The drawing under review shows one solid part. Ordinate dimensions are in mm from its lowest x, y, z. A direction names the side the tool comes from. Give positions to 0.01 mm unless a question says otherwise; leave off trailing zeros. Loops run counter-clockwise (first coordinate to the right, second up) from the corner with the lowest first, then second, coordinate; pieces in that order, holes last. Notation, with made-up numbers: M -7,63.5 L 39,63.5 A26 ccw 39,80.5 Z; hole C -2.5,63 d6. An arc over 180 degrees is marked long. Answer as CSV lines item,"result".
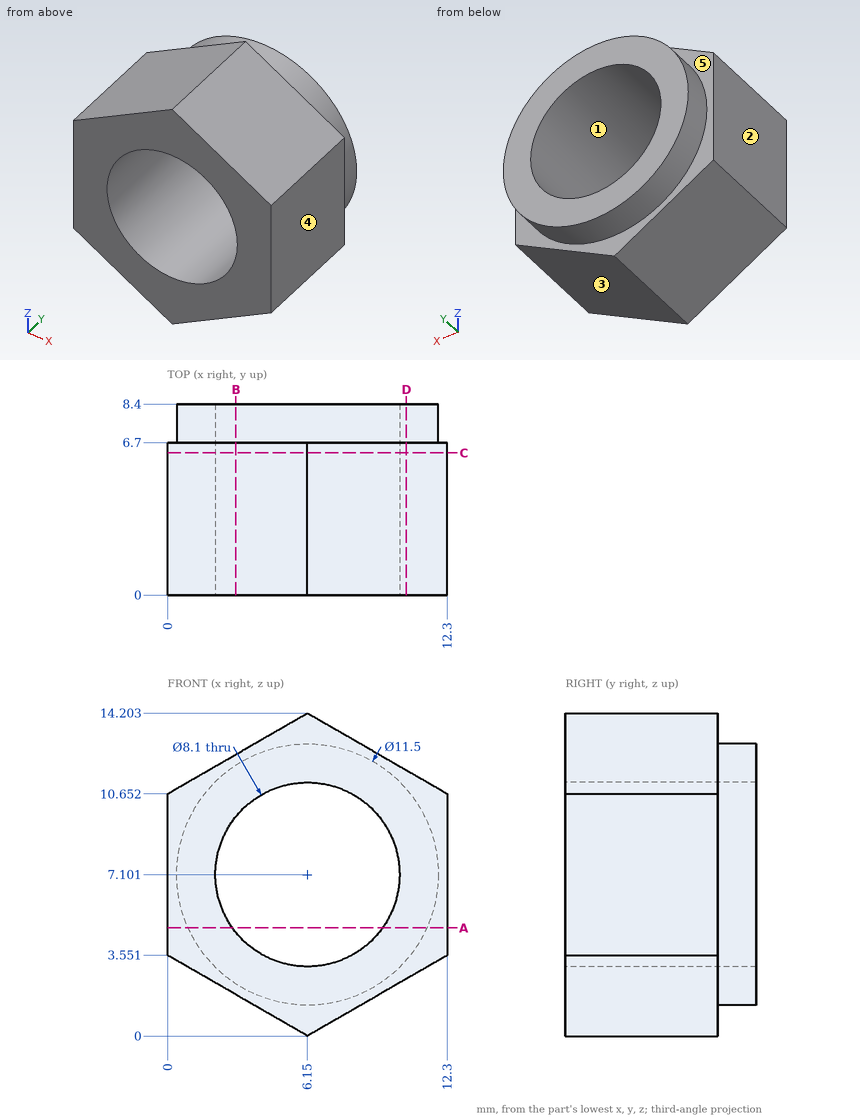
1. We need section B-B, the plane x = 3. Write out the cut boundary in (y, z) (1 decimal).
Answer block:
outline,"M 0,1.8 L 6.7,1.8 L 6.7,2.3 L 8.4,2.3 L 8.4,4.6 L 0,4.6 Z; M 0,9.6 L 8.4,9.6 L 8.4,11.9 L 6.7,11.9 L 6.7,12.4 L 0,12.4 Z"
2. We need section A-A, the plane z = 4.75. Write out the cut boundary in (x, y).
Answer block:
outline,"M 0,0 L 2.85,0 L 2.85,8.4 L 0.9,8.4 L 0.9,6.7 L 0,6.7 Z; M 9.45,0 L 12.3,0 L 12.3,6.7 L 11.4,6.7 L 11.4,8.4 L 9.45,8.4 Z"
3. We need section C-C, the plane y = 6.25. Write out the cut boundary in (x, z).
Answer block:
outline,"M 0,3.55 L 6.15,0 L 12.3,3.55 L 12.3,10.65 L 6.15,14.2 L 0,10.65 Z; hole C 6.15,7.1 d8.1"
4. The part is to be moulded in two halves that separate along X. For the marked faces 1, 2 and 3, say which applies: pulls with the +X half, pulls with the -X half, needs draft (parallel to the pull), parting line crosses it, or undercut.
Answer block:
face 1,"undercut"
face 2,"pulls with the -X half"
face 3,"pulls with the +X half"
5. We need section D-D, the plane x = 10.5. Write out the cut boundary in (y, z), plus the area to 3 significant figures.
Answer block:
outline,"M 0,2.51 L 6.7,2.51 L 6.7,3.34 L 8.4,3.34 L 8.4,10.86 L 6.7,10.86 L 6.7,11.69 L 0,11.69 Z"
area,"74.3 mm²"
6. To check wall thickness, follow L1, parallel to X at y = 6.5, z = 7.25; L2, parallel to Y at x = 4.5, z = 1.5; L3, parallel to Z at x = 8.75, y = 5 (1 decimal). State the ranges of each line that lie inside material, in increasing order. Write a range as [from, to].
Answer block:
L1,"[0, 2.1], [10.2, 12.3]"
L2,"[0, 6.7]"
L3,"[1.5, 4], [10.2, 12.7]"
7. For the marked faces 4 and 5, list the 3-axis set-ups (+Z, -Z, +X, -X, +Y, -Y) from which the entire face can be reached by the end or side of a thin tool; tool diameter is ignored.
Answer block:
face 4,"+Z, -Z, +X, +Y, -Y"
face 5,"+Y"
8. For P1, Ø6.5, axis at x = 6.15, z = 7.1, coming from the +Y side, flat-tipped, find the tip position at first contact; note if it passes through.
Answer block:
P1,"through"
